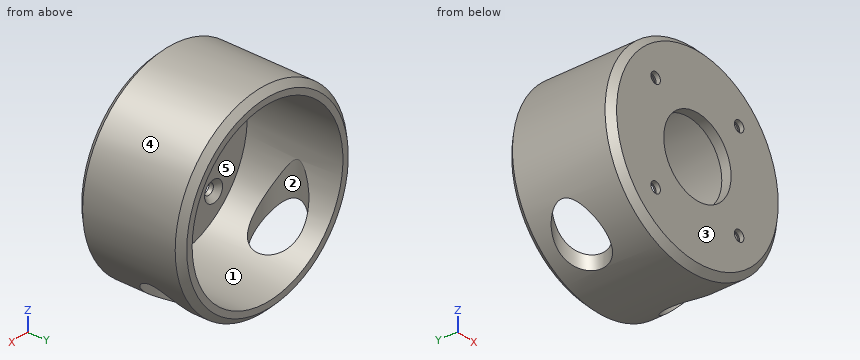
from build123d import *

# Parameters (mm, degrees)
SKETCH2_R           = 32
SKETCH2_R_2         = 28
BOSS_EXTRUDE1_DEPTH = 34
SKETCH3_R           = 28
BOSS_EXTRUDE2_DEPTH = 3
SKETCH4_R           = 12.5
CUT_EXTRUDE1_DEPTH  = 3
SKETCH5_R           = 2.6
SKETCH5_R_2         = 1.75
CUT_EXTRUDE2_DEPTH  = 4
CHAMFER1_SIZE       = 1.6
CHAMFER2_SIZE       = 2
CHAMFER3_SIZE       = 2
SKETCH7_R           = 7.5
CUT_EXTRUDE4_DEPTH  = 33


with BuildPart() as part:
    # Sketch2 → Boss-Extrude1 (new body)
    with BuildSketch(Plane(origin=(0, 0, 0), x_dir=(1, 0, 0), z_dir=(0, 1, 0))):
        Circle(SKETCH2_R)
        Circle(SKETCH2_R_2, mode=Mode.SUBTRACT)
    extrude(amount=BOSS_EXTRUDE1_DEPTH)

    # Sketch3 → Boss-Extrude2 (add)
    with BuildSketch(Plane.XZ):
        Circle(SKETCH3_R)
    extrude(amount=-BOSS_EXTRUDE2_DEPTH)

    # Sketch4 → Cut-Extrude1 (cut)
    with BuildSketch(Plane(origin=(0, 3, 0), x_dir=(1, 0, 0), z_dir=(0, 1, 0))):
        Circle(SKETCH4_R)
    extrude(amount=-CUT_EXTRUDE1_DEPTH, mode=Mode.SUBTRACT)

    # Sketch5 → Cut-Extrude2 (cut, through all)
    with BuildSketch(Plane(origin=(0, 3, 0), x_dir=(1, 0, 0), z_dir=(0, 1, 0))):
        Circle(SKETCH5_R)
        with Locations((-15.5, 15.5)):
            Circle(SKETCH5_R_2)
        with Locations((15.5, 15.5)):
            Circle(SKETCH5_R_2)
        with Locations((-15.5, -15.5)):
            Circle(SKETCH5_R_2)
        with Locations((15.5, -15.5)):
            Circle(SKETCH5_R_2)
    extrude(amount=-CUT_EXTRUDE2_DEPTH, mode=Mode.SUBTRACT)

    # Chamfer1
    chamfer1_edges = [part.edges().sort_by_distance(p)[0] for p in [
        (13.75, 3, 15.5),
        (-17.25, 3, 15.5),
        (13.75, 3, -15.5),
        (-17.25, 3, -15.5),
    ]]
    chamfer(chamfer1_edges, length=CHAMFER1_SIZE)

    # Chamfer2
    chamfer2_edges = [part.edges().sort_by_distance(p)[0] for p in [
        (-32, 0, 0),
    ]]
    chamfer(chamfer2_edges, length=CHAMFER2_SIZE)

    # Chamfer3
    chamfer3_edges = [part.edges().sort_by_distance(p)[0] for p in [
        (-32, 34, 0),
    ]]
    chamfer(chamfer3_edges, length=CHAMFER3_SIZE)

    # Sketch7 → Cut-Extrude4 (cut, through all)
    with BuildSketch(Plane.XY):
        with Locations((-20, 20)):
            Circle(SKETCH7_R)
        with Locations((20, 20)):
            Circle(SKETCH7_R)
    extrude(amount=-CUT_EXTRUDE4_DEPTH, mode=Mode.SUBTRACT)


solid = part.part
Model file for the job. Use its own axes, mm. Face numbers are marked on the shaded views. A direction names the side the tool comes from. Give positions to 0.01 mm unless a question says otherwise; leave off trailing zeros. Order: outer loops, then holes, each group sorted by start corner. A loop starts at its lowest first (then second) coordinate and runs counter-clockwise, first axis right, second up. Notation, with made-up numbers: M 38,19 L 55,19 A16 cw 55,46 Z; hole C -27.5,-24 d6. An arc over 180 degrees is marked long. Put each result on its own line as item: value. Start each with the question number.
(1) Band-saw the part on A-A on z = 0. Give the cut face in (x, y).
(2) Pull direction Z, two halves, no side cores. Call the marked faces 3, 4 and 5: released by +Z, released by -Z, zero draft, split by the parting line, or undercut.
(3) Pin check, flat tips, straight feed: pin 1 Ø1 at (x, y) = (3, 3.5) entering from -Z; pin 2 Ø19.5 at (x, y) = (20, 20) entering from -Z; pin 3 Ø5 at (x, y) = (-0.5, 20.5) entering from +Z. Stop position of each tip, or through.
(4) Band-saw the part on B-B on y = 16. Give the cut face in (x, z).
(5) Band-saw the part on D-D on y = 20. Give the cut face in (x, z).
(6) Band-saw the part on C-C on x = -15. Count the separate pieces of the cut face and the enclosed holes in it, then the cut area to 3 significant figures.
(7) Tool access for the marked faces 1 and 2: list every direction of +Z, -Z, +X, -X, +Y, -Y with a clear straight run to the whole face (end or side of a thin tool).
(8) Drill centre lines: L1, parallel to Z at x = 15.5, y = 1; L2, parallel to Z at x = -15.5, y = 0.8; L3, parallel to X at y = 0.6, z = 15.5. Where is each one in solid material? Low to high. Write a range as [from, to].
Results below:
1. outline: M -32,2 L -30,0 L -12.5,0 L -12.5,3 L -28,3 L -28,34 L -30,34 L -32,32 Z; M 12.5,0 L 30,0 L 32,2 L 32,32 L 30,34 L 28,34 L 28,3 L 12.5,3 Z
2. face 3: zero draft
2. face 4: split by the parting line
2. face 5: undercut
3. pin 1: stops at z = -31.9
3. pin 2: stops at z = -30.31
3. pin 3: stops at z = 32
4. outline: M -26.34,-18.17 L -26.34,-9.49 A28 cw long 26.34,-9.49 L 26.34,-18.17 A32 ccw long Z; M -13.66,-28.94 A32 ccw 13.66,-28.94 L 13.66,-24.44 A28 cw -13.66,-24.44 Z
5. outline: M -27.5,-16.36 L -27.5,-5.27 A28 cw long 27.5,-5.27 L 27.5,-16.36 A32 ccw long Z; M -12.5,-29.46 A32 ccw 12.5,-29.46 L 12.5,-25.05 A28 cw -12.5,-25.05 Z
6. separate pieces: 4
6. enclosed holes: 0
6. area: 370 mm2
7. face 1: +Y
7. face 2: -Z
8. L1: z = [-26.85, -17.25], [-13.75, 13.75], [17.25, 26.85]
8. L2: z = [-26.62, -17.25], [-13.75, 13.75], [17.25, 26.62]
8. L3: x = [-26.38, -17.25], [-13.75, 13.75], [17.25, 26.38]
